from build123d import *

# Parameters (mm, degrees)
F0_R     = 9
F1_DEPTH = 17
F2_DEPTH = 10.5
F4_DEPTH = 1.5


# Not quite as in the source:
# - a feature names something its author has since deleted; it is built from what else it names


with BuildPart() as f1:
    # F0 (on Top) → F1 (new body)
    with BuildSketch(Plane.XY):
        Circle(F0_R)
        with BuildLine():
            ThreePointArc((-2.7, 3.3466401061), (1.8547236991, 3.8794329483), (4.3, 0))
            ThreePointArc((4.3, 0), (1.8547236991, -3.8794329483), (-2.7, -3.3466401061))
            ThreePointArc((-2.7, -3.3466401061), (-4.3, 0), (-2.7, 3.3466401061))
        make_face(mode=Mode.SUBTRACT)
        with BuildLine():
            ThreePointArc((-2.7, -3.3466401061), (1.8547236991, -3.8794329483), (4.3, 0))
            ThreePointArc((4.3, 0), (1.8547236991, 3.8794329483), (-2.7, 3.3466401061))
            Line((-2.7, 3.3466401061), (-2.7, -3.3466401061))
        make_face()
        with BuildLine():
            Line((-1.7, -2.8284271247), (-1.7, 2.8284271247))
            ThreePointArc((-1.7, 2.8284271247), (3.3, 0), (-1.7, -2.8284271247))
        make_face(mode=Mode.SUBTRACT)
        with BuildLine():
            ThreePointArc((-1.7, -2.8284271247), (3.3, 0), (-1.7, 2.8284271247))
            Line((-1.7, 2.8284271247), (-1.7, -2.8284271247))
        make_face()
        with BuildLine():
            Line((-2.7, -3.3466401061), (-2.7, 3.3466401061))
            ThreePointArc((-2.7, 3.3466401061), (-4.3, 0), (-2.7, -3.3466401061))
        make_face()
    extrude(amount=F1_DEPTH)

    # F0 (on Top) → F2 (join)
    with BuildSketch(Plane.XY):
        with BuildLine():
            ThreePointArc((-2.7, -3.3466401061), (1.8547236991, -3.8794329483), (4.3, 0))
            ThreePointArc((4.3, 0), (1.8547236991, 3.8794329483), (-2.7, 3.3466401061))
            Line((-2.7, 3.3466401061), (-2.7, -3.3466401061))
        make_face()
        with BuildLine():
            Line((-1.7, -2.8284271247), (-1.7, 2.8284271247))
            ThreePointArc((-1.7, 2.8284271247), (3.3, 0), (-1.7, -2.8284271247))
        make_face(mode=Mode.SUBTRACT)
    extrude(amount=-F2_DEPTH)

    # F3 (on face) → F4 (join)
    with BuildSketch(Plane.XY.offset(17)):
        Polygon((-1.5, -7.5), (0, -9), (1.5, -7.5), (1.5, -0.5), (-1.5, -0.5), align=None)
    extrude(amount=F4_DEPTH)


solid = f1.part
Design review of the part built by this model. Coordinates are the model's own, in mm. A direction names the side the tool comes from. Round coordinates to 2 decimals unless told otherwise and drop trailing zeros. Write each loop counter-clockwise with the first axis right and the second up, starting at its lowest first coordinate (ties: lowest second). Pieces come first, ordered by that corner, then holes.
Item 1: Consider section D-D on y = -1.25. Give the boundary of the cut face in (x, z), and give its area (3 significant figures).
Item 2: Consider section A-A on y = -4.75. Give the boundary of the cut face in (x, z).
Item 3: For pin 1 Ø5 at (x, z) = (1.5, -4) entering from -Y; pin 2 Ø5.5 at (y, z) = (0.5, -6.5) entering from -X; pin 3 Ø1.2 at (x, z) = (-0.5, 18) entering from +Y, all flat-tipped, find the tip position at first contact; note any pin that passes through.
Item 4: Consider section C-C on x = 4.75. Give the boundary of the cut face in (y, z).
Item 5: For faces 5 (the flat face through (0, -0.5, 18)), 6 (the flat face through (-2.7, 0, -5)), 7 (the flat face through (-1.5, -4, 18)), 8 (the flat face through (1, -8, 18)), 9 (the flat face through (-1.7, 0, -5)), list the 3-axis set-ups (+Z, -Z, +X, -X, +Y, -Y) from which the entire face can be reached by the end or side of a thin tool; tool diameter is ignored.
Item 6: Draft analysis for pull direction X (two halves, no side actions). For faces 1 (the cylindrical face through (3.3, 0.1, -5.2)), 2 (the flat face through (-1, -8, 18)), 3 (the flat face through (1.5, -4, 18)), 4 (the flat face through (0, -5, 18.5)), state which applies: released by +X, released by -X, zero draft, split by the parting line, or undercut.
Item 7: Consider section B-B on z = 6.5. Give the boundary of the cut face in (x, y), and give its area (3 significant figures).
Item 8: Wall thickness on L1, parallel to Y at x = 0, z = -8.5; L2, parallel to Z at x = 6.5, y = -5.5; L3, parallel to X at y = -3, z = 13.25: over which ranges is each line inside the solid? List them lowest first.
Check values:
1. outline: (-8.91, 0) - (-2.7, 0) - (-2.7, -10.5) - (-1.7, -10.5) - (-1.7, 0) - (3.05, 0) - (3.05, -10.5) - (4.11, -10.5) - (4.11, 0) - (8.91, 0) - (8.91, 17) - (1.5, 17) - (1.5, 18.5) - (-1.5, 18.5) - (-1.5, 17) - (-8.91, 17) - close
1. area: 329 mm2
2. outline: (-7.64, 0) - (7.64, 0) - (7.64, 17) - (1.5, 17) - (1.5, 18.5) - (-1.5, 18.5) - (-1.5, 17) - (-7.64, 17) - close
3. pin 1: stops at y = -4.3
3. pin 2: stops at x = -2.7
3. pin 3: stops at y = -0.5
4. outline: (-7.64, 0) - (7.64, 0) - (7.64, 17) - (-7.64, 17) - close
5. face 5: +Z, +X, -X, +Y
5. face 6: -Z, -X, +Y, -Y
5. face 7: +Z, -X, +Y, -Y
5. face 8: +Z, +X, -Y
5. face 9: -Z
6. face 1: undercut
6. face 2: released by -X
6. face 3: released by +X
6. face 4: zero draft
7. outline: circle Ø18 at (0, 0)
7. area: 254 mm2
8. L1: y = -4.3 to -3.3, 3.3 to 4.3
8. L2: z = 0 to 17
8. L3: x = -8.49 to 8.49
